For this review, take the finished solid that the model builds, in its own axes (mm). Coordinates: 2 decimals unless noted, no trailing zeros. Order: outer loops, then holes, each group sorted by start corner. A loop starts at its lowest first (then second) coordinate and runs counter-clockwise, first axis right, second up. Notation, with made-up numbers: M 23,48.5 L 29,48.5 A31 ccw 29,87.5 Z; hole C 80,5 d3. An arc over 180 degrees is marked long. Use CSV: the item, a comma, the result in double quotes.
```python
from build123d import *

# Parameters (mm, degrees)
SKETCH_1_R          = 2
EXTRUDE_1_DEPTH     = 3
CUT_EXTRUDE_1_DEPTH = 3


with BuildPart() as part:
    # ｽｹｯﾁ1 → ﾎﾞｽ - 押し出し1 (new body)
    with BuildSketch(Plane(origin=(0, 0, 0), x_dir=(0, 0, -1), z_dir=(1, 0, 0))):
        with BuildLine():
            Line((75.819108386, -1.462182475), (70.301486023, -23.420893584))
            ThreePointArc((70.301486023, -23.420893584), (71.18795254, -30.585212423), (76.666666667, -35.285954792))
            ThreePointArc((76.666666667, -35.285954792), (79.927992798, -40.845509894), (75, -45))
            Line((75, -45), (-5, -45))
            ThreePointArc((-5, -45), (-9.927992798, -40.845509894), (-6.666666667, -35.285954792))
            ThreePointArc((-6.666666667, -35.285954792), (-1.303429587, -30.794428268), (-0.196130789, -23.88704006))
            Line((-0.196130789, -23.88704006), (-4.803895914, -0.965703915))
            ThreePointArc((-4.803895914, -0.965703915), (-2.920865081, 3.934278482), (2.314364214, 4.318995055))
            Line((2.314364214, 4.318995055), (23.261645602, -6.905754637))
            ThreePointArc((23.261645602, -6.905754637), (35.593052242, -9.845509438), (47.770153464, -6.320746485))
            Line((47.770153464, -6.320746485), (66.916984028, 5.14733062))
            ThreePointArc((66.916984028, 5.14733062), (73.576725635, 4.817367926), (75.819108386, -1.462182475))
        make_face()
        Circle(SKETCH_1_R, mode=Mode.SUBTRACT)
        with Locations((70, 0)):
            Circle(SKETCH_1_R, mode=Mode.SUBTRACT)
        with Locations((-5, -40)):
            Circle(SKETCH_1_R, mode=Mode.SUBTRACT)
        with Locations((75, -40)):
            Circle(SKETCH_1_R, mode=Mode.SUBTRACT)
        with Locations((10, -40)):
            Circle(SKETCH_1_R, mode=Mode.SUBTRACT)
        with Locations(Location((60, -40, 0), (0, 0, 180))):
            Circle(SKETCH_1_R, mode=Mode.SUBTRACT)
    extrude(amount=EXTRUDE_1_DEPTH)

    # ｽｹｯﾁ4 → ｶｯﾄ - 押し出し1 (cut)
    with BuildSketch(Plane(origin=(3, 0, 0), x_dir=(0, 0, -1), z_dir=(1, 0, 0))):
        with BuildLine():
            Line((16.388456854, -17.18013778), (23.759978506, -30.003236627))
            ThreePointArc((23.759978506, -30.003236627), (23.75717928, -32.001617006), (22.026063059, -33))
            Line((22.026063059, -33), (13.442662844, -33))
            ThreePointArc((13.442662844, -33), (11.884294691, -32.253590323), (11.489107607, -30.571488698))
            ThreePointArc((11.489107607, -30.571488698), (11.999153131, -26.050896834), (11.568512265, -21.52205088))
            Line((11.568512265, -21.52205088), (10.767826216, -17.539036649))
            ThreePointArc((10.767826216, -17.539036649), (11.53641023, -15.539043834), (13.673238513, -15.382016661))
            Line((13.673238513, -15.382016661), (15.599179861, -16.414046028))
            ThreePointArc((15.599179861, -16.414046028), (16.047519114, -16.74176593), (16.388456854, -17.18013778))
        make_face()
        with BuildLine():
            Line((26.191058921, -24.199740762), (30.673276651, -31.996763373))
            ThreePointArc((30.673276651, -31.996763373), (31.405575092, -32.731116222), (32.407192098, -33))
            Line((32.407192098, -33), (37.592807902, -33))
            ThreePointArc((37.592807902, -33), (38.594424908, -32.731116222), (39.326723349, -31.996763373))
            Line((39.326723349, -31.996763373), (43.808941079, -24.199740762))
            ThreePointArc((43.808941079, -24.199740762), (43.707310227, -22.047275438), (41.710827194, -21.236417067))
            ThreePointArc((41.710827194, -21.236417067), (35, -21.852586388), (28.289172806, -21.236417067))
            ThreePointArc((28.289172806, -21.236417067), (26.292689773, -22.047275438), (26.191058921, -24.199740762))
        make_face()
        with BuildLine():
            Line((58.663269251, -20.496528634), (59.471345903, -17.280592385))
            ThreePointArc((59.471345903, -17.280592385), (58.723884986, -15.187408917), (56.503971117, -15.077421353))
            Line((56.503971117, -15.077421353), (54.382909172, -16.347840593))
            ThreePointArc((54.382909172, -16.347840593), (53.983753774, -16.662131254), (53.676665716, -17.066854093))
            Line((53.676665716, -17.066854093), (46.240021494, -30.003236627))
            ThreePointArc((46.240021494, -30.003236627), (46.24282072, -32.001617006), (47.973936941, -33))
            Line((47.973936941, -33), (56.557337156, -33))
            ThreePointArc((56.557337156, -33), (58.115705309, -32.253590323), (58.510892393, -30.571488698))
            ThreePointArc((58.510892393, -30.571488698), (58.002515762, -25.52516752), (58.663269251, -20.496528634))
        make_face()
    extrude(amount=-CUT_EXTRUDE_1_DEPTH, mode=Mode.SUBTRACT)


solid = part.part
```
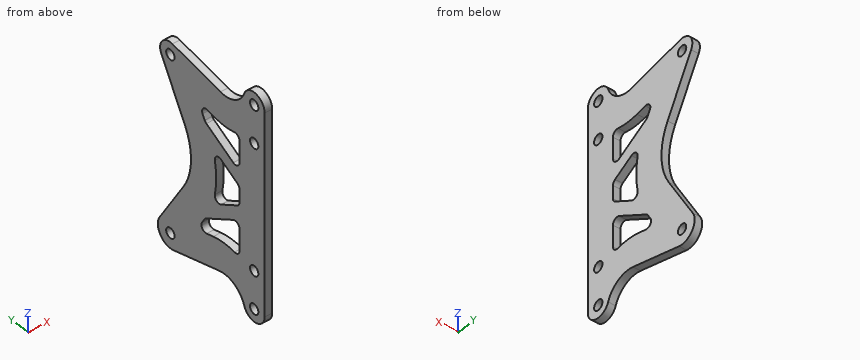
Item 1: Add section B-B on y = 0. State the section outline as (x, z) points, and give its area (3 significant figures).
Solutions:
outline,"M 0,-76 L 3,-76 L 3,-72 L 0,-72 Z; M 0,-68 L 3,-68 L 3,-58.32 L 0,-58.32 Z; M 0,-10.37 L 3,-10.37 L 3,-2 L 0,-2 Z; M 0,2 L 3,2 L 3,4.9 L 0,4.9 Z"
area,"74.9 mm^2"
Item 2: Clearance check with flat-ended pins moving along their axes: pin 1 Ø1.5 at (x, y) = (2, -34) entering from +Z; pin 2 Ø1.5 at (x, z) = (1, -54) entering from +Y. State where each tip first meets the part, or that it passes through.
Solutions:
pin 1,"z = 5.43"
pin 2,"y = -2.14"
Item 3: To check wall thickness, follow line 1 along Z through (x, y) = (1.85, -31); line 2 along Y through (x, z) = (1.65, -10); line 3 along Z through (x, y) = (2.25, -24.5). State the ranges of each line that lie inside material, in increasing order. Write a range as [from, to].
Solutions:
line 1,"[-71.42, -58.56], [-45.97, -39.9], [-30.1, -24.03], [-11.44, 1.42]"
line 2,"[-45, -42], [-38, 0.2]"
line 3,"[-70.09, -58.04], [-49.4, -43.64], [-26.36, -20.6], [-11.96, 0.09]"
Item 4: Add section A-A on y = -40. State the section outline as (x, z) points.
Solutions:
outline,"M 0,-80 L 3,-80 L 3,-77 L 0,-77 Z; M 0,-73 L 3,-73 L 3,-62 L 0,-62 Z; M 0,-58 L 3,-58 L 3,-12 L 0,-12 Z; M 0,-8 L 3,-8 L 3,3 L 0,3 Z; M 0,7 L 3,7 L 3,10 L 0,10 Z"
Item 5: Add section C-C on x = 1.4. State how many separate pieces and enclosed holes the cut face has, and give its area (3 significant figures).
Solutions:
separate pieces,"1"
enclosed holes,"9"
area,"2,780 mm^2"
Item 6: Add section D-D on y = -11. State the section outline as (x, z) points.
Solutions:
outline,"M 0,-73.42 L 3,-73.42 L 3,2.79 L 0,2.79 Z"
